```python
from build123d import *

# Parameters (mm, degrees)
SKETCH1_R           = 4
BOSS_EXTRUDE1_DEPTH = 1.5
FILLET3_R           = 15


with BuildPart() as part:
    # Sketch1 → Boss-Extrude1 (new, symmetric)
    with BuildSketch(Plane.XY):
        with BuildLine():
            Line((-2, 5.656854249), (-2, 22.630988629))
            Line((-2, 22.630988629), (-11.030624508, 39.078825188))
            ThreePointArc((-11.030624508, 39.078825188), (-14.887660916, 50.259411986), (-7.524349851, 41.003932465))
            Line((-7.524349851, 41.003932465), (2, 23.656854249))
            Line((2, 23.656854249), (2, 5.656854249))
            ThreePointArc((2, 5.656854249), (0, -6), (-2, 5.656854249))
        make_face()
        Circle(SKETCH1_R, mode=Mode.SUBTRACT)
        with Locations((-12, 45)):
            Circle(SKETCH1_R, mode=Mode.SUBTRACT)
    extrude(amount=BOSS_EXTRUDE1_DEPTH, both=True)

    # Fillet3
    fillet3_edges = [part.edges().sort_by_distance(p)[0] for p in [
        (-2, 5.656854249, 0),
        (-2, 22.630988629, 0),
        (-11.030624508, 39.078825188, 0),
        (-7.524349851, 41.003932465, 0),
        (2, 23.656854249, 0),
        (2, 5.656854249, 0),
    ]]
    fillet(fillet3_edges, radius=FILLET3_R)


solid = part.part
```
The listing builds one solid part. Answer for the finished solid, in the listing's coordinates (mm). A direction names the side the tool comes from. Give positions to 0.01 mm unless a question says otherwise; leave off trailing zeros. Write each loop counter-clockwise with the first axis right and the second up, starting at its lowest first coordinate (ties: lowest second). Pieces come first, ordered by that corner, then holes. Notation, with made-up numbers: M 3.25,88 L 12.25,88 A16 cw 12.25,98 Z; hole C 29,71 d7. An arc over 180 degrees is marked long. Write each question's results on one line, items separated by ' | '.
Q1. Section C-C, the plane x = 3 is taken. Write down the section's boundary in (y, z).
Output values:
outline: M -5.2,-1.5 L -2.65,-1.5 L -2.65,1.5 L -5.2,1.5 Z; M 2.65,-1.5 L 6.94,-1.5 L 6.94,1.5 L 2.65,1.5 Z
Q2. Section B-B, the plane x = -3.25 is taken. Write down the section's boundary in (y, z).
Output values:
outline: M -5.04,-1.5 L -2.33,-1.5 L -2.33,1.5 L -5.04,1.5 Z; M 2.33,-1.5 L 6.33,-1.5 L 6.33,1.5 L 2.33,1.5 Z; M 24.78,-1.5 L 33.22,-1.5 L 33.22,1.5 L 24.78,1.5 Z
Q3. Consider L1, parallel to Y at x = -12, z = -0.45; L2, parallel to Y at x = 0, z = 0.5; L3, parallel to X at y = 42, z = 0.85. Determine where each line is inside the solid, lowest interval first. Write a range as from..to.
Output values:
L1: 38.04..41, 49..51 | L2: -6..-4, 4..27.3 | L3: -17.2..-14.65, -9.35..-6.16
Q4. Flat-ended cylindrical pins translate along their axes: P1, Ø0.9, axis at y = 14.5, z = 0, coming from the +X side; P2, Ø12, axis at x = 3, y = 40.5, coming from the -Z side; P3, Ø1, axis at x = -6, z = -0.5, coming from the -Y side; P4, Ø1.5, axis at y = 17, z = -0.5, coming from the -X side. Find the tip coordinate at first contact, or state that the pin passes through.
Output values:
P1: x = 2 | P2: through | P3: y = -2.4 | P4: x = -2
Q5. A tool of negligible diameter and unlimited length cuts with its end or side. For faces 1 (the flat face through (-5.81, 29.57, 0.02)), 2 (the flat face through (2, 16, 0)), 3 (the cylindrical face through (0, -6, 0)), from which of +Z, -Z, +X, -X, +Y, -Y can it reach the whole face along a straight path? Write none if from no direction.
Output values:
face 1: +Z, -Z, -X | face 2: +Z, -Z, +X, +Y | face 3: +Z, -Z
Q6. Section D-D, the plane z = 0.1 is taken. Write down the section's boundary in (x, y), then the cut area to 3 significant figures.
Output values:
outline: M -14.56,39.57 A15 cw -7.82,33.23 L -3.85,26 A15 cw -2,18.78 L -2,12.33 A15 cw -4.86,3.52 A6 ccw long 4.86,3.52 A15 cw 2,12.33 L 2,19.81 A15 ccw 0.15,27.03 L -4.31,35.16 A15 cw -6.05,44.25 A6 ccw long Z; hole C -12,45 d8; hole C 0,0 d8 | area: 288 mm2
Q7. Section A-A, the plane y = 45 is taken. Write down the section's boundary in (x, z), then the cut area to 3 significant figures.
Output values:
outline: M -18,-1.5 L -16,-1.5 L -16,1.5 L -18,1.5 Z; M -8,-1.5 L -6,-1.5 L -6,1.5 L -8,1.5 Z | area: 12.0 mm2
Q8. For a pull along Y with two mould halves and no side action, classify faces 4 (the flat face through (-2, 23, 1.5)), 5 (the cylindrical face through (-5.887, 39.501, -0.021)), 6 (the cylindrical face through (-2.7, 7.8, 0)), 7 (the cylindrical face through (1.517, 23.587, 0.021)) as released by +Y, released by -Y, zero draft, split by the parting line, or undercut.
Output values:
face 4: zero draft | face 5: undercut | face 6: undercut | face 7: released by +Y
